For this review, use the dimensioned drawing (mm, ordinates from the lowest corner) and the shaded views. Coordinates: 2 decimals unless noted, no trailing zeros. Order: outer loops, then holes, each group sorted by start corner. A loop starts at its lowest first (then second) coordinate and runs counter-clockwise, first axis right, second up. Notation, with made-up numbers: (-22, 30.25) -> (-3, 30.25) arc R17 cw to (-3, 46.25) -> close; hole circle Ø5 at (88, 43.5). An arc over 180 degrees is marked (long way). Use CSV: the item, a comma, the result in double quotes. Start each with the question number.
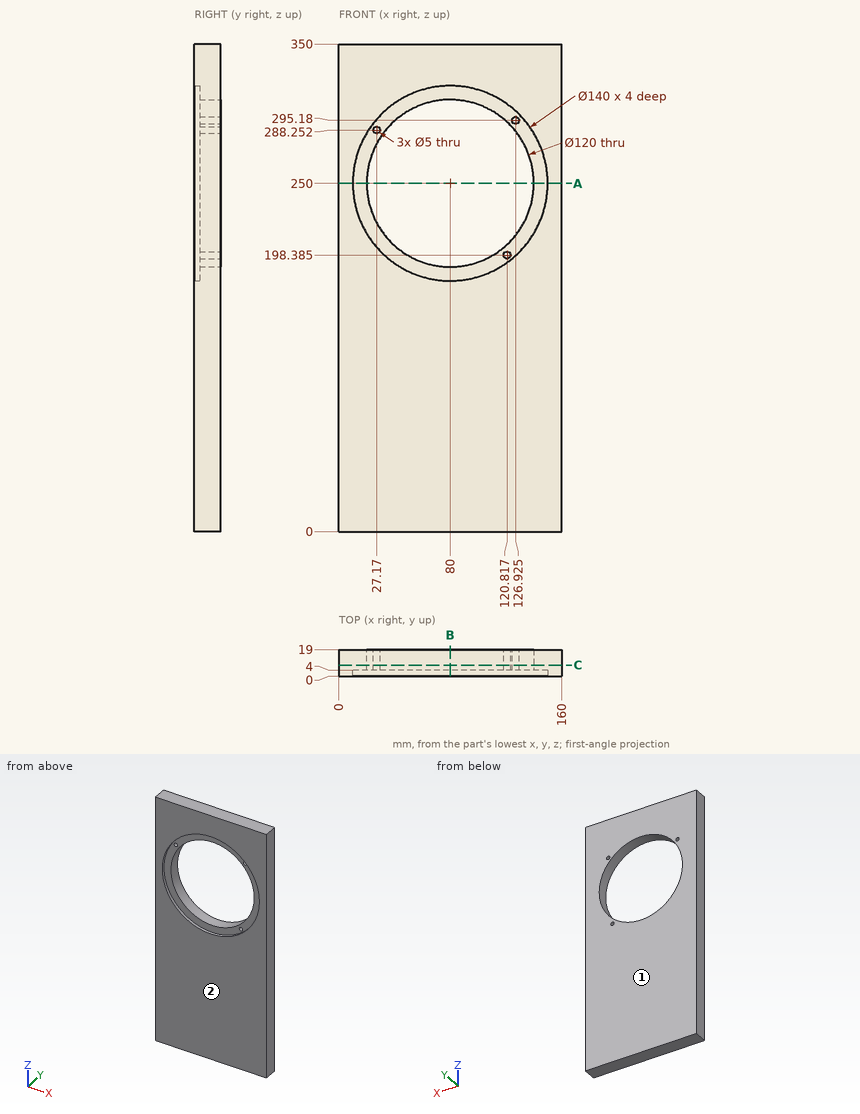
Q1. Draft analysis for pull direction Y (two halves, no side actions). For the marked faces 1 and 2, state which applies: +Y half, -Y half, draft (parallel to the pull), parting line (faces both ways), or undercut.
Q2. Add section C-C, the plane y = 7.75. State the section outline as (x, z) points (1 decimal).
Q3. Add section A-A, the plane z = 250. State the section outline as (x, y) points, then the cut area to 3 significant figures.
Q4. Clearance check with a flat-ended pin moving along its axis: pin 1 Ø8 at (x, z) = (120.82, 198.38) entering from -Y. State where the tip first meets the part, or that it passes through.
Q5. To check wall thickness, follow probe 1 along Z at (x, y) = (80, 8.5); probe 2 along Z at (x, y) = (82, 1); probe 3 along X at (y, z) = (3.5, 272.5) (1 decimal). State the ranges of each line that lie inside material, in increasing order.
Q6. Add section B-B, the plane x = 80. State the section outline as (y, z) points, then the cut area to 3 significant figures.
Answer block:
1,face 1,"+Y half"
1,face 2,"-Y half"
2,outline,"(0, 0) -> (160, 0) -> (160, 350) -> (0, 350) -> close; hole circle Ø120 at (80, 250); hole circle Ø5 at (27.2, 288.3); hole circle Ø5 at (120.8, 198.4); hole circle Ø5 at (126.9, 295.2)"
3,outline,"(0, 0) -> (10, 0) -> (10, 4) -> (20, 4) -> (20, 19) -> (0, 19) -> close; (140, 4) -> (150, 4) -> (150, 0) -> (160, 0) -> (160, 19) -> (140, 19) -> close"
3,area,"680 mm²"
4,pin 1,"stops at y = 4"
5,probe 1,"z = 0 to 190, 310 to 350"
5,probe 2,"z = 0 to 180.03, 319.97 to 350"
5,probe 3,"x = 0 to 13.7, 146.3 to 160"
6,outline,"(0, 0) -> (19, 0) -> (19, 190) -> (4, 190) -> (4, 180) -> (0, 180) -> close; (0, 320) -> (4, 320) -> (4, 310) -> (19, 310) -> (19, 350) -> (0, 350) -> close"
6,area,"4,290 mm²"
